from build123d import *

# Parameters (mm, degrees)
SKETCH1_R           = 4.5
BOSS_EXTRUDE1_DEPTH = 0.8
SKETCH2_R           = 4
BOSS_EXTRUDE2_DEPTH = 2.5
SKETCH3_R           = 1.5
CUT_EXTRUDE1_DEPTH  = 12.5


with BuildPart() as part:
    # Sketch1 → Boss-Extrude1 (new body)
    with BuildSketch(Plane(origin=(0, 0, 0), x_dir=(1, 0, 0), z_dir=(0, 1, 0))):
        with Locations(Location((0, 0, 0), (0, 0, 270))):
            Circle(SKETCH1_R)
    extrude(amount=BOSS_EXTRUDE1_DEPTH)

    # Sketch2 → Boss-Extrude2 (add)
    with BuildSketch(Plane(origin=(0, 0.8, 0), x_dir=(-1, 0, 0), z_dir=(0, -1, 0))):
        with Locations(Location((0, 0, 0), (0, 0, 180))):
            Circle(SKETCH2_R)
    extrude(amount=-BOSS_EXTRUDE2_DEPTH)

    # Sketch3 → Cut-Extrude1 (cut)
    with BuildSketch(Plane(origin=(0, 0, 0), x_dir=(1, 0, 0), z_dir=(0, 1, 0))):
        with Locations(Location((0, 0, 0), (0, 0, 90))):
            Circle(SKETCH3_R)
    extrude(amount=CUT_EXTRUDE1_DEPTH, mode=Mode.SUBTRACT)


solid = part.part
Work out the finished part from the listing and answer in its coordinate system (mm). A direction names the side the tool comes from. Give positions to 0.01 mm unless a question says otherwise; leave off trailing zeros. Write each loop counter-clockwise with the first axis right and the second up, starting at its lowest first coordinate (ties: lowest second). Pieces come first, ordered by that corner, then holes. Notation, with made-up numbers: (49, 82.5) - (101, 82.5) arc R21 cw to (101, 102.5) - close; hole circle Ø4 at (10.5, 16). An arc over 180 degrees is marked (long way). One line per item, written item: value. Start each with the question number.
1. Find section B-B (z = 0). Write down the section's boundary in (x, y), then the cut area to 3 significant figures.
2. For faces 1 (the cylindrical face through (-0.45, 1.63, -1.43)), 2 (the flat face through (-3, 0.8, -3)), determine the directions among +Z, -Z, +X, -X, +Y, -Y from which every point of the face is accessible in a straight line to the end or side of a thin tool.
3. Find section C-C (y = 1.65). Write down the section's boundary in (x, z).
4. Find section D-D (z = -1.75). Write down the section's boundary in (x, y).
5. Find section A-A (x = 0). Write down the section's boundary in (y, z).
6. Consider probe 1 along Z at (x, y) = (-1.25, 0.3); probe 2 along Z at (x, y) = (1, 1.25). Determine where each line is inside the solid, lowest interval first.
Geometry results:
1. outline: (-4.5, 0) - (-1.5, 0) - (-1.5, 3.3) - (-4, 3.3) - (-4, 0.8) - (-4.5, 0.8) - close; (1.5, 0) - (4.5, 0) - (4.5, 0.8) - (4, 0.8) - (4, 3.3) - (1.5, 3.3) - close
1. area: 17.3 mm2
2. face 1: +Y, -Y
2. face 2: +Y
3. outline: circle Ø8 at (0, 0); hole circle Ø3 at (0, 0)
4. outline: (-4.15, 0) - (4.15, 0) - (4.15, 0.8) - (3.6, 0.8) - (3.6, 3.3) - (-3.6, 3.3) - (-3.6, 0.8) - (-4.15, 0.8) - close
5. outline: (0, -4.5) - (0.8, -4.5) - (0.8, -4) - (3.3, -4) - (3.3, -1.5) - (0, -1.5) - close; (0, 1.5) - (3.3, 1.5) - (3.3, 4) - (0.8, 4) - (0.8, 4.5) - (0, 4.5) - close
6. probe 1: -4.32 to -0.83, 0.83 to 4.32
6. probe 2: -3.87 to -1.12, 1.12 to 3.87
